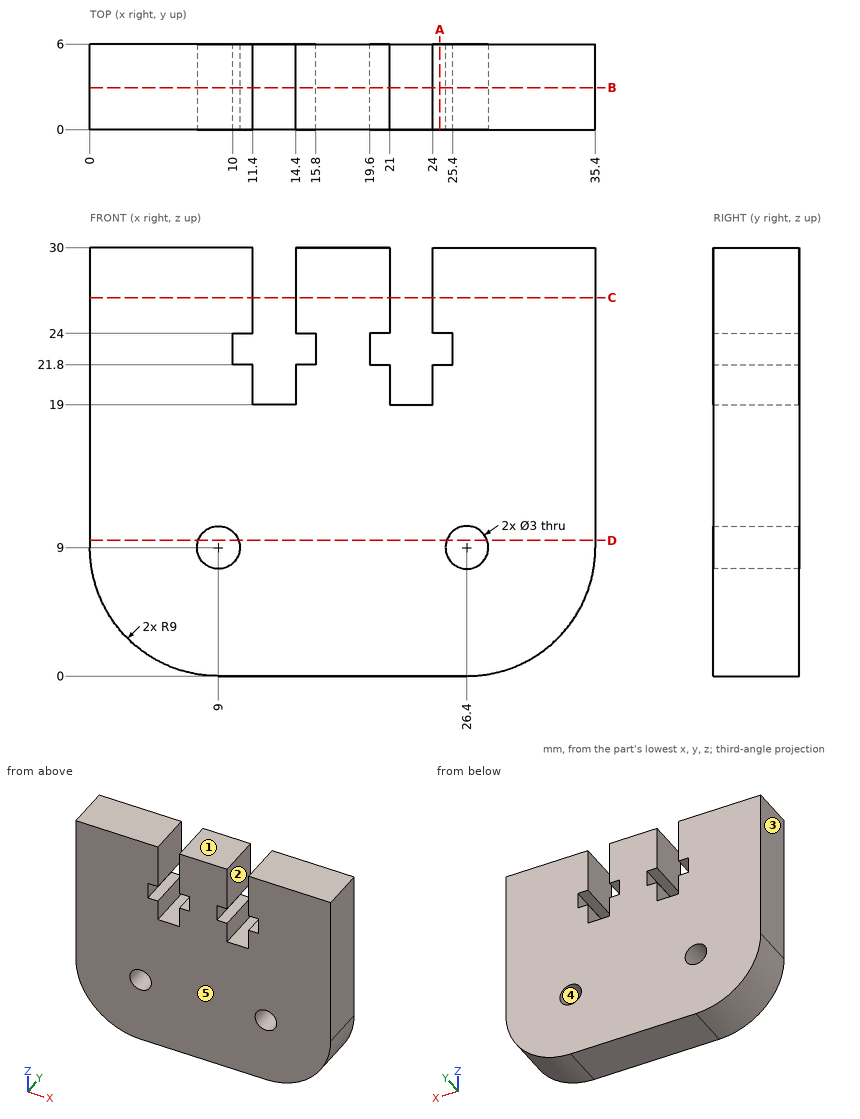
Check sheet for the drawn part. Datum: minimum x, y, z corner. Units: mm. A direction names the side the tool comes from. Round coordinates to 2 decimals unless told otherwise and drop trailing zeros. Loops run counter-clockwise (first coordinate to the right, second up) from the corner with the lowest first, then second, coordinate; pieces in that order, holes last. Notation, with made-up numbers: (-17.75, -33) -> (14.25, -33) arc R17 ccw to (14.25, -5) -> close; hole circle Ø1 at (-40, -2.75). An arc over 180 degrees is marked (long way). Put each result on its own line as item: value. Start each with the question number.
1. Section check D-D (z = 9.5). Enter the section's corners in (x, y).
2. Section check A-A (x = 24.5). Enter the section's corners in (y, z).
3. Section check C-C (z = 26.5). Enter the section's corners in (x, y), plus the area to 3 significant figures.
4. Gauge pin test, flat ends, axial feed: pin 1 (0.9 mm diameter, centred on x = 13.5, y = 3, fed in from +Z); pin 2 (2.5 mm diameter, centred on x = 26.4, z = 9, fed in from +Y). Record the tip position at first contact, or that the pin passes through.
5. Access from +Z, -Z, +X, -X, +Y, -Y to the whole of each face (thin tool, end or side, straight path). Record for the marked faces 1 and 2.
6. Scan lines: probe 1 along X at (y, z) = (3.65, 24.25); probe 2 along X at (y, z) = (3.4, 9); probe 3 along Z at (x, y) = (23.5, 3.05). Record each from-to range of solid material in increasing order.
7. Section check B-B (y = 2.95). Give the number of separate pieces and of enclosed holes in the cut face, plus the area to 3 significant figures.
8. Draft check along X on the marked faces 3, 4 and 5. Enter one of: +X half, -X half, draft (parallel to the pull), parting line (faces both ways), or undercut.
Findings:
1. outline: (0, 0) -> (7.59, 0) -> (7.59, 6) -> (0, 6) -> close; (10.41, 0) -> (24.99, 0) -> (24.99, 6) -> (10.41, 6) -> close; (27.81, 0) -> (35.4, 0) -> (35.4, 6) -> (27.81, 6) -> close
2. outline: (0, 0) -> (6, 0) -> (6, 21.8) -> (0, 21.8) -> close; (0, 24) -> (6, 24) -> (6, 30) -> (0, 30) -> close
3. outline: (0, 0) -> (11.4, 0) -> (11.4, 6) -> (0, 6) -> close; (14.4, 0) -> (21, 0) -> (21, 6) -> (14.4, 6) -> close; (24, 0) -> (35.4, 0) -> (35.4, 6) -> (24, 6) -> close
3. area: 176 mm^2
4. pin 1: stops at z = 19
4. pin 2: passes through
5. face 1: +Z, +X, -X, +Y, -Y
5. face 2: +Z, +Y, -Y
6. probe 1: x = 0 to 11.4, 14.4 to 21, 24 to 35.4
6. probe 2: x = 0 to 7.5, 10.5 to 24.9, 27.9 to 35.4
6. probe 3: z = 0 to 19
7. separate pieces: 1
7. enclosed holes: 2
7. area: 935 mm^2
8. face 3: -X half
8. face 4: undercut
8. face 5: draft
